Geometry check sheet. Reference: the model listing, model coordinates, mm. A direction names the side the tool comes from. Round coordinates to 2 decimals unless told otherwise and drop trailing zeros. Write each loop counter-clockwise with the first axis right and the second up, starting at its lowest first coordinate (ties: lowest second). Pieces come first, ordered by that corner, then holes. Notation, with made-up numbers: (-5.5, 15) - (38.5, 15) arc R20 ccw to (38.5, 21) - close; hole circle Ø4 at (17.5, -5.5). An arc over 180 degrees is marked (long way). Return JSON: item names as keys, results as strings.
```python
from build123d import *

# Parameters (mm, degrees)
SKETCH2_R           = 4.91
SKETCH2_R_2         = 3.91
BOSS_EXTRUDE1_DEPTH = 13.8
BOSS_EXTRUDE2_DEPTH = 13.8


with BuildPart() as part:
    # Sketch2 → Boss-Extrude1 (new body)
    with BuildSketch(Plane(origin=(0, 0, 0), x_dir=(1, 0, 0), z_dir=(0, 1, 0))):
        Circle(SKETCH2_R)
        Circle(SKETCH2_R_2, mode=Mode.SUBTRACT)
    extrude(amount=BOSS_EXTRUDE1_DEPTH)

    # Sketch3 → Boss-Extrude2 (add)
    with BuildSketch(Plane(origin=(0, 13.8, 0), x_dir=(1, 0, 0), z_dir=(0, 1, 0))):
        with BuildLine():
            Line((4.785195921, 1.1), (10.185195921, 1.1))
            Line((10.185195921, 1.1), (10.185195921, 2.1))
            Line((10.185195921, 2.1), (10.785195921, 2.1))
            Line((10.785195921, 2.1), (10.785195921, -2.1))
            Line((10.785195921, -2.1), (10.185195921, -2.1))
            Line((10.185195921, -2.1), (10.185195921, -1.1))
            Line((10.185195921, -1.1), (4.785195921, -1.1))
            ThreePointArc((4.785195921, -1.1), (4.91, 0), (4.785195921, 1.1))
        make_face()
        with BuildLine():
            Line((4.694101229, -1.439970016), (9.37063841, -4.139970016))
            Line((9.37063841, -4.139970016), (9.87063841, -3.273944612))
            Line((9.87063841, -3.273944612), (10.390253652, -3.573944612))
            Line((10.390253652, -3.573944612), (8.290253652, -7.211251308))
            Line((8.290253652, -7.211251308), (7.77063841, -6.911251308))
            Line((7.77063841, -6.911251308), (8.27063841, -6.045225905))
            Line((8.27063841, -6.045225905), (3.594101229, -3.345225905))
            ThreePointArc((3.594101229, -3.345225905), (4.252184733, -2.455), (4.694101229, -1.439970016))
        make_face()
        with BuildLine():
            Line((3.345225905, -3.594101229), (6.045225905, -8.27063841))
            Line((6.045225905, -8.27063841), (6.911251308, -7.77063841))
            Line((6.911251308, -7.77063841), (7.211251308, -8.290253652))
            Line((7.211251308, -8.290253652), (3.573944612, -10.390253652))
            Line((3.573944612, -10.390253652), (3.273944612, -9.87063841))
            Line((3.273944612, -9.87063841), (4.139970016, -9.37063841))
            Line((4.139970016, -9.37063841), (1.439970016, -4.694101229))
            ThreePointArc((1.439970016, -4.694101229), (2.455, -4.252184733), (3.345225905, -3.594101229))
        make_face()
        with BuildLine():
            Line((1.1, -4.785195921), (1.1, -10.185195921))
            Line((1.1, -10.185195921), (2.1, -10.185195921))
            Line((2.1, -10.185195921), (2.1, -10.785195921))
            Line((2.1, -10.785195921), (-2.1, -10.785195921))
            Line((-2.1, -10.785195921), (-2.1, -10.185195921))
            Line((-2.1, -10.185195921), (-1.1, -10.185195921))
            Line((-1.1, -10.185195921), (-1.1, -4.785195921))
            ThreePointArc((-1.1, -4.785195921), (0, -4.91), (1.1, -4.785195921))
        make_face()
        with BuildLine():
            Line((-1.439970016, -4.694101229), (-4.139970016, -9.37063841))
            Line((-4.139970016, -9.37063841), (-3.273944612, -9.87063841))
            Line((-3.273944612, -9.87063841), (-3.573944612, -10.390253652))
            Line((-3.573944612, -10.390253652), (-7.211251308, -8.290253652))
            Line((-7.211251308, -8.290253652), (-6.911251308, -7.77063841))
            Line((-6.911251308, -7.77063841), (-6.045225905, -8.27063841))
            Line((-6.045225905, -8.27063841), (-3.345225905, -3.594101229))
            ThreePointArc((-3.345225905, -3.594101229), (-2.455, -4.252184733), (-1.439970016, -4.694101229))
        make_face()
        with BuildLine():
            Line((-3.594101229, -3.345225905), (-8.27063841, -6.045225905))
            Line((-8.27063841, -6.045225905), (-7.77063841, -6.911251308))
            Line((-7.77063841, -6.911251308), (-8.290253652, -7.211251308))
            Line((-8.290253652, -7.211251308), (-10.390253652, -3.573944612))
            Line((-10.390253652, -3.573944612), (-9.87063841, -3.273944612))
            Line((-9.87063841, -3.273944612), (-9.37063841, -4.139970016))
            Line((-9.37063841, -4.139970016), (-4.694101229, -1.439970016))
            ThreePointArc((-4.694101229, -1.439970016), (-4.252184733, -2.455), (-3.594101229, -3.345225905))
        make_face()
        with BuildLine():
            Line((-4.785195921, -1.1), (-10.185195921, -1.1))
            Line((-10.185195921, -1.1), (-10.185195921, -2.1))
            Line((-10.185195921, -2.1), (-10.785195921, -2.1))
            Line((-10.785195921, -2.1), (-10.785195921, 2.1))
            Line((-10.785195921, 2.1), (-10.185195921, 2.1))
            Line((-10.185195921, 2.1), (-10.185195921, 1.1))
            Line((-10.185195921, 1.1), (-4.785195921, 1.1))
            ThreePointArc((-4.785195921, 1.1), (-4.91, 0), (-4.785195921, -1.1))
        make_face()
        with BuildLine():
            Line((-4.694101229, 1.439970016), (-9.37063841, 4.139970016))
            Line((-9.37063841, 4.139970016), (-9.87063841, 3.273944612))
            Line((-9.87063841, 3.273944612), (-10.390253652, 3.573944612))
            Line((-10.390253652, 3.573944612), (-8.290253652, 7.211251308))
            Line((-8.290253652, 7.211251308), (-7.77063841, 6.911251308))
            Line((-7.77063841, 6.911251308), (-8.27063841, 6.045225905))
            Line((-8.27063841, 6.045225905), (-3.594101229, 3.345225905))
            ThreePointArc((-3.594101229, 3.345225905), (-4.252184733, 2.455), (-4.694101229, 1.439970016))
        make_face()
        with BuildLine():
            Line((-3.345225905, 3.594101229), (-6.045225905, 8.27063841))
            Line((-6.045225905, 8.27063841), (-6.911251308, 7.77063841))
            Line((-6.911251308, 7.77063841), (-7.211251308, 8.290253652))
            Line((-7.211251308, 8.290253652), (-3.573944612, 10.390253652))
            Line((-3.573944612, 10.390253652), (-3.273944612, 9.87063841))
            Line((-3.273944612, 9.87063841), (-4.139970016, 9.37063841))
            Line((-4.139970016, 9.37063841), (-1.439970016, 4.694101229))
            ThreePointArc((-1.439970016, 4.694101229), (-2.455, 4.252184733), (-3.345225905, 3.594101229))
        make_face()
        with BuildLine():
            Line((-1.1, 4.785195921), (-1.1, 10.185195921))
            Line((-1.1, 10.185195921), (-2.1, 10.185195921))
            Line((-2.1, 10.185195921), (-2.1, 10.785195921))
            Line((-2.1, 10.785195921), (2.1, 10.785195921))
            Line((2.1, 10.785195921), (2.1, 10.185195921))
            Line((2.1, 10.185195921), (1.1, 10.185195921))
            Line((1.1, 10.185195921), (1.1, 4.785195921))
            ThreePointArc((1.1, 4.785195921), (0, 4.91), (-1.1, 4.785195921))
        make_face()
        with BuildLine():
            Line((1.439970016, 4.694101229), (4.139970016, 9.37063841))
            Line((4.139970016, 9.37063841), (3.273944612, 9.87063841))
            Line((3.273944612, 9.87063841), (3.573944612, 10.390253652))
            Line((3.573944612, 10.390253652), (7.211251308, 8.290253652))
            Line((7.211251308, 8.290253652), (6.911251308, 7.77063841))
            Line((6.911251308, 7.77063841), (6.045225905, 8.27063841))
            Line((6.045225905, 8.27063841), (3.345225905, 3.594101229))
            ThreePointArc((3.345225905, 3.594101229), (2.455, 4.252184733), (1.439970016, 4.694101229))
        make_face()
        with BuildLine():
            Line((3.594101229, 3.345225905), (8.27063841, 6.045225905))
            Line((8.27063841, 6.045225905), (7.77063841, 6.911251308))
            Line((7.77063841, 6.911251308), (8.290253652, 7.211251308))
            Line((8.290253652, 7.211251308), (10.390253652, 3.573944612))
            Line((10.390253652, 3.573944612), (9.87063841, 3.273944612))
            Line((9.87063841, 3.273944612), (9.37063841, 4.139970016))
            Line((9.37063841, 4.139970016), (4.694101229, 1.439970016))
            ThreePointArc((4.694101229, 1.439970016), (4.252184733, 2.455), (3.594101229, 3.345225905))
        make_face()
    extrude(amount=-BOSS_EXTRUDE2_DEPTH)


solid = part.part
```
(1) Release check for a two-part mould opening along Z. For faces 3 (the face through (-2.77, 7, 7)), 4 (the face through (-9.355, 6.997, -5.367)), 5 (the face through (-5.367, 6.997, 9.355)) record: pulls with the +Z half, pulls with the -Z half, needs draft (parallel to the pull), parting line crosses it, or undercut.
Response values:
{"face 3": "undercut", "face 4": "pulls with the -Z half", "face 5": "pulls with the +Z half"}
(2) Material ranges on line 1 along X through (y, z) = (10.75, 0); line 2 along Z through (x, y) = (-9.25, 9.75); line 3 along X through (y, z) = (4.25, 7.5), recorded low to high. Write a range as [from, to].
Response values:
{"line 1": "x = [-10.79, -3.91], [3.91, 10.79]", "line 2": "z = [-5.55, -4.07], [-1.1, 1.1], [4.07, 5.55]", "line 3": "x = [-5.6, -3.06], [-1.1, 1.1], [3.06, 5.6]"}
(3) Access from +Z, -Z, +X, -X, +Y, -Y to the whole of each face (thin tool, end or side, straight path). Record for faces 1 (the face through (9.355, 6.997, 5.367)), 2 (the face through (9.62, 7, 3.71)).
Response values:
{"face 1": "+Z, +X, +Y, -Y", "face 2": "+Y, -Y"}
(4) Section check B-B, the plane x = 0. Enter the section's corners in (y, z), plus the area to 3 significant figures.
Response values:
{"outline": "(0, -10.79) - (13.8, -10.79) - (13.8, -3.91) - (0, -3.91) - close; (0, 3.91) - (13.8, 3.91) - (13.8, 10.79) - (0, 10.79) - close", "area": "190 mm^2"}
(5) Section check A-A, the plane z = 0. Enter the section's corners in (x, y).
Response values:
{"outline": "(-10.79, 0) - (-3.91, 0) - (-3.91, 13.8) - (-10.79, 13.8) - close; (3.91, 0) - (10.79, 0) - (10.79, 13.8) - (3.91, 13.8) - close"}
(6) Gauge pin test, flat ends, axial feed: pin 1 (7 mm diameter, centred on x = 0, z = 0, fed in from -Y); pin 2 (3 mm diameter, centred on y = 11, z = -4.5, fed in from -X); pin 3 (0.5 mm diameter, centred on y = 9, z = 10.5, fed in from -X); pin 4 (4 mm diameter, centred on y = 5, z = 3, fed in from -X). Record the tip position at first contact, or that the pin passes through.
Response values:
{"pin 1": "passes through", "pin 2": "stops at x = -10.39", "pin 3": "stops at x = -3.82", "pin 4": "stops at x = -10.79"}
